```python
from build123d import *

# Parameters (mm, degrees)
SKETCH1_R           = 12
BOSS_EXTRUDE1_DEPTH = 33.53
CUT_EXTRUDE1_DEPTH  = 19.6
CHAMFER1_SIZE       = 0.4
SKETCH3_R           = 9.375
CUT_EXTRUDE2_DEPTH  = 3.4
CUT_EXTRUDE2_DRAFT  = -35
SKETCH4_W           = 24
SKETCH4_H           = 14.42225279
CUT_EXTRUDE3_DEPTH  = 17.4
SKETCH5_R           = 2.415
CUT_EXTRUDE4_DEPTH  = 33.7
SCALE1_SCALE        = 0.49


with BuildPart() as part:
    # Sketch1 → Boss-Extrude1 (new body)
    with BuildSketch(Plane(origin=(0, 0, 0), x_dir=(1, 0, 0), z_dir=(0, 1, 0))):
        with Locations(Location((0, 0, 0), (0, 0, 270))):
            Circle(SKETCH1_R)
    extrude(amount=BOSS_EXTRUDE1_DEPTH)

    # Sketch2 → Cut-Extrude1 (cut)
    with BuildSketch(Plane(origin=(0, 33.53, 0), x_dir=(1, 0, 0), z_dir=(0, 1, 0))):
        with BuildLine():
            Line((-6.5, 6.5), (-2.5, 6.5))
            ThreePointArc((-2.5, 6.5), (0, 7.211126395), (2.5, 6.5))
            Line((2.5, 6.5), (6.5, 6.5))
            Line((6.5, 6.5), (6.5, 2.5))
            ThreePointArc((6.5, 2.5), (7.211126395, 0), (6.5, -2.5))
            Line((6.5, -2.5), (6.5, -6.5))
            Line((6.5, -6.5), (2.5, -6.5))
            ThreePointArc((2.5, -6.5), (0, -7.211126395), (-2.5, -6.5))
            Line((-2.5, -6.5), (-6.5, -6.5))
            Line((-6.5, -6.5), (-6.5, -2.5))
            ThreePointArc((-6.5, -2.5), (-7.211126395, 0), (-6.5, 2.5))
            Line((-6.5, 2.5), (-6.5, 6.5))
        make_face()
    extrude(amount=-CUT_EXTRUDE1_DEPTH, mode=Mode.SUBTRACT)

    # Chamfer1
    chamfer1_edges = [part.edges().sort_by_distance(p)[0] for p in [
        (-6.5, 23.73, -6.5),
        (6.5, 23.73, -6.5),
        (6.5, 23.73, 6.5),
        (-6.5, 23.73, 6.5),
    ]]
    chamfer(chamfer1_edges, length=CHAMFER1_SIZE)


with BuildPart() as cut_extrude2_tool:
    # Sketch3 → Cut-Extrude2 (with draft: the straight prism first)
    with BuildSketch(Plane(origin=(0, 33.53, 0), x_dir=(1, 0, 0), z_dir=(0, 1, 0))):
        Circle(SKETCH3_R)
    extrude(amount=-CUT_EXTRUDE2_DEPTH)
    # Cut-Extrude2: the draft: its side faces are tilted about the plane it starts from
    cut_extrude2_sides = [cut_extrude2_tool.faces().sort_by_distance(p)[0] for p in [
        (-9.375, 31.83, 0),
    ]]
    draft(cut_extrude2_sides, Plane(origin=(0, 33.53, 0), x_dir=(1, 0, 0), z_dir=(0, 1, 0)), CUT_EXTRUDE2_DRAFT)


with BuildPart() as part_1:
    add(part.part)

    # Cut-Extrude2: cut by cut_extrude2_tool
    add(cut_extrude2_tool.part, mode=Mode.SUBTRACT)

    # Sketch4 → Cut-Extrude3 (cut)
    with BuildSketch(Plane.XZ):
        Rectangle(SKETCH4_W, SKETCH4_H)
    extrude(amount=-CUT_EXTRUDE3_DEPTH, mode=Mode.SUBTRACT)

    # Sketch5 → Cut-Extrude4 (cut, symmetric)
    with BuildSketch(Plane.XY):
        with Locations(Location((0, 7, 0), (0, 0, 90))):
            Circle(SKETCH5_R)
        with BuildLine():
            ThreePointArc((-6.854820161, 5.581747356), (0, 0), (6.854820161, 5.581747356))
            Line((6.854820161, 5.581747356), (9.3, 17.4))
            Line((9.3, 17.4), (12, 17.4))
            Line((12, 17.4), (12, -3.192277431))
            Line((12, -3.192277431), (-12, -3.192277431))
            Line((-12, -3.192277431), (-12, 17.4))
            Line((-12, 17.4), (-9.3, 17.4))
            Line((-9.3, 17.4), (-6.854820161, 5.581747356))
        make_face()
    extrude(amount=CUT_EXTRUDE4_DEPTH, both=True, mode=Mode.SUBTRACT)


with BuildPart() as part_2:
    # Scale1: scaled about (-1.86e-07, 20.712300737, 4.053e-06)
    add(part_1.part.scale(SCALE1_SCALE).moved(Location((-9.5e-08, 10.563273376, 2.067e-06))))


solid = part_2.part
```
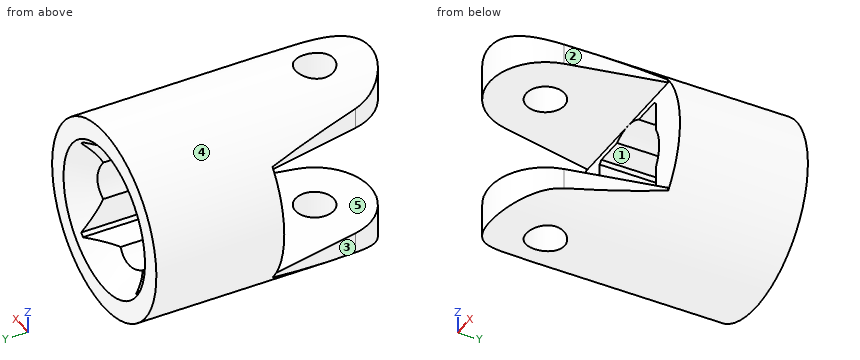
The listing builds one solid part. Answer for the finished solid, in the listing's coordinates (mm). Face numbers are marked on the shaded views. A direction names the side the tool comes from. Give positions to 0.01 mm unless a question says otherwise; leave off trailing zeros. Order: outer loops, then holes, each group sorted by start corner. A loop starts at its lowest first (then second) coordinate and runs counter-clockwise, first axis right, second up. Notation, with made-up numbers: (-38, -22.75) -> (-11, -22.75) arc R31 ccw to (-11, 9.25) -> close; hole circle Ø4 at (14.5, 32). An arc over 180 degrees is marked (long way). Answer as CSV lines item,"result". Start each with the question number.
Q1. Determine the mould class of the marked faces 3, 4 and 5 for opening direction Z: pulls with the +Z half, pulls with the -Z half, needs draft (parallel to the pull), parting line crosses it, or undercut.
Q2. Which of the six approach directions +Z, -Z, +X, -X, +Y, -Y give full straight-line access (tool end or side, diameter ignored) to the marked faces 1 and 2?
Q3. Find the intervals of material crossed by L1, parallel to Y at x = 0, z = 5.1; L2, parallel to Z at x = -4.5, y = 19; L3, parallel to Y at x = 0, z = -4.5, in increasing order.
Q4. A cutting plane is placed at B-B (y = 14.5). Determine the outline of the cut face in (x, z), then the cut area to 3 significant figures.
Q5. A cutting plane is placed at A-A (y = 12.25). Determine the outline of the cut face in (x, z).
Q6. Given pin 1 (0.5 mm diameter, centred on x = 2, y = 21.5, fed in from +Z); pin 2 (5 mm diameter, centred on x = 0, z = 1.5, fed in from +Y) (3 decimals); pin 3 (2 mm diameter, centred on x = 3.5, y = 23, fed in from -Z), each flat-ended and moving along its own axis, determine where each tip first touches the part or whether it passes through.
Results found:
1,face 3,"needs draft"
1,face 4,"parting line crosses it"
1,face 5,"undercut"
2,face 1,"+Y, -Y"
2,face 2,"+Z, -Z, +X, -Y"
3,L1,"10.56 to 12.81, 15.18 to 26.99"
3,L2,"-3.78 to -3.53, 3.53 to 3.78"
3,L3,"10.56 to 12.81, 15.18 to 26.86"
4,outline,"(-3.61, -4.64) arc R5.88 ccw to (-1.07, -5.78) -> (-1.07, -3.53) -> (-3.61, -3.53) -> close; (-3.61, 3.53) -> (-1.07, 3.53) -> (-1.07, 5.78) arc R5.88 ccw to (-3.61, 4.64) -> close; (1.07, -5.78) arc R5.88 ccw to (3.61, -4.64) -> (3.61, -3.53) -> (1.07, -3.53) -> close; (1.07, 3.53) -> (3.61, 3.53) -> (3.61, 4.64) arc R5.88 ccw to (1.07, 5.78) -> close"
4,area,"18.3 mm2"
5,outline,"(-2.95, -5.08) arc R5.88 ccw to (2.95, -5.08) -> (2.95, -3.53) -> (-2.95, -3.53) -> close; (-2.95, 3.53) -> (2.95, 3.53) -> (2.95, 5.08) arc R5.88 ccw to (-2.95, 5.08) -> close"
6,pin 1,"z = 5.61"
6,pin 2,"y = 26.145"
6,pin 3,"z = -5.32"
